Work out the finished part from the listing and answer in its coordinate system (mm). Face numbers are marked on the shaded views. Coordinates: 2 decimals unless noted, no trailing zeros. Order: outer loops, then holes, each group sorted by start corner. A loop starts at its lowest first (then second) coordinate and runs counter-clockwise, first axis right, second up. Notation, with made-up numbers: M 47.5,12 L 59.5,12 A20 ccw 59.5,17 Z; hole C -0.75,86.25 d8. An arc over 180 degrees is marked long. Write item = value, one per line. Start each with the question number.
Q1. Each of these flat-tipped pins is pushed along its axis until it touches: P1, Ø1.5, axis at x = -8, y = 4, coming from the -Z side; P2, Ø3, axis at x = -9.5, y = 2, coming from the -Z side. Where does it stop, or does it pass through?
Q2. Find section A-A on y = 3.5. Give the vertices of the cut face in (x, z) (3 decimals).
Q3. Straight lines are drawn through the part: line 1 along Z through (x, y) = (0, 8.2); line 2 along X through (y, z) = (4, -0.5); line 3 along Z through (x, y) = (0, 0.85). For each, find the intervals that lie inside material, in ascending order.
Q4. Find section D-D on z = 24. Give the vertices of the cut face in (x, y), and give its area (3 significant figures).
Q5. Determine the mould class of the marked faces 1, 2 and 3 for opening direction X: released by +X, released by -X, zero draft, split by the parting line, or undercut.
Q6. Find section B-B on z = 0. Give the vertices of the cut face in (x, y), and give its area (4 significant figures).
Q7. Find section C-C on x = -22.5. Give the vertices of the cut face in (y, z), and give its area (3 significant figures).
Autodesk Inventor part; units mm, degrees
ref_plane "YZ Plane" through (0, 0, 0) normal (1, 0, 0) x (0, 1, 0)
ref_plane "XZ Plane" through (0, 0, 0) normal (0, 1, 0) x (-1, 0, 0)
ref_plane "XY Plane" through (0, 0, 0) normal (0, 0, 1) x (1, 0, 0)
sketch "Náčrt1" plane through (0, 0, 0) normal (0, 1, 0) x (-1, 0, 0)
  line L0 (0, -49) -> (0, 49)
  line L1 (35, -35) -> (-35, -35)
  line L2 (-35, -35) -> (-35, 35)
  line L3 (-35, 35) -> (35, 35)
  line L4 (35, 35) -> (35, -35)
  line L5 (-49, 0) -> (49, 0)
  dimension "d9" = 70
  dimension "d10" = 70
extrude "Vysunutí1" add sketch "Náčrt1" along normal blind 10
fillet "Zaoblení1" radius 6 2 edges at (35, 5, -35) (-35, 5, 35)
fillet "Zaoblení2" radius 34 1 edges at (-35, 5, -35)
sketch "Náčrt2" plane through (0, 10, 0) normal (0, 1, 0) x (1, 0, 0)
  line L0 (0, 49) -> (0, -49)
  line L1 (49, 0) -> (-49, 0)
  point P0 (0, 0)
  point P1 (0, 0)
hole "Díra1" at (0, 10, 0) direction (0, -1, 0) diameter 60.1 depth 7.3 counterbore diameter 62.9 counterbore depth 5.1
sketch "Náčrt3" plane through (0, 2.7, 0) normal (0, 1, 0) x (1, 0, 0)
  line L0 (0, 49) -> (0, -49)
  line L1 (49, 0) -> (-49, 0)
  point P0 (0, 0)
  point P1 (0, 0)
hole "Díra2" at (0, 2.7, 0) direction (0, -1, 0) diameter 58.2 end through all
sketch "Náčrt4" plane through (0, 10, 0) normal (0, 1, 0) x (1, 0, 0)
  arc A0 (-35, -29) -> (-29, -35) centre (-29, -29) ccw
  arc A1 (35, 29) -> (29, 35) centre (29, 29) ccw
  point P0 (0, 0)
hole "Díra3" at (-29, 10, 29) at (29, 10, -29) direction (0, -1, 0) diameter 3.9 end through all
sketch "Náčrt5" plane through (0, 10, 0) normal (0, 1, 0) x (1, 0, 0)
  arc A0 (17.5, -30.3109) -> (30.3109, -17.5) centre (0, 0) ccw
  line L0 (0, 49) -> (0, -49)
  line L1 (49, 0) -> (-49, 0)
  line L2 (0, 0) -> (17.5, -30.3109)
  line L3 (30.3109, -17.5) -> (0, 0)
  dimension "d35" = 35
  dimension "d36" = 30
  dimension "d37" = 30
extrude "Vysunutí2" cut sketch "Náčrt5" against normal up to surface (10 mm away)
fillet "Zaoblení4" radius 20 1 edges at (35, 5, 35)
properties part number "4.L - GM - 01.03" material "LCP plast"
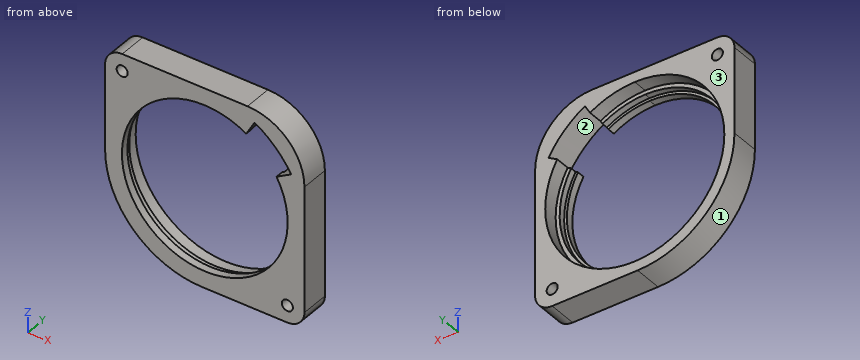
Findings below:
q1.P1 = -34.42
q1.P2 = -34.27
q2.outline = M -35,-1 A34 ccw -1,-35 L 29,-35 A6 ccw 35,-29 L 35,15 A20 ccw 15,35 L -29,35 A6 ccw -35,29 Z; hole C -29,29 d3.9; hole M 15.025,26.024 A30.05 ccw long 26.024,15.025 L 30.311,17.5 A35 ccw 17.5,30.311 Z; hole C 29,-29 d3.9
q3.line_1 = -35 to -31.45, 31.45 to 35
q3.line_2 = -35 to -30.05, 30.05 to 35
q3.line_3 = -35 to -29.1, 29.1 to 35
q4.outline = M -35,0 L -16.46,0 L -16.46,2.7 L -18.08,2.7 L -18.08,4.9 L -20.32,4.9 L -20.32,10 L -35,10 Z; M 25.48,0 L 32.86,0 L 32.86,10 L 25.48,10 Z
q4.area = 236 mm^2
q5.face_1 = released by -X
q5.face_2 = undercut
q5.face_3 = zero draft
q6.outline = M -35,0 L -29.1,0 L -29.1,2.7 L -30.05,2.7 L -30.05,4.9 L -31.45,4.9 L -31.45,10 L -35,10 Z; M 29.1,0 L 35,0 L 35,10 L 31.45,10 L 31.45,4.9 L 30.05,4.9 L 30.05,2.7 L 29.1,2.7 Z
q6.area = 89.85 mm^2
q7.outline = M 0,-27.34 L 10,-27.34 L 10,-21.97 L 4.9,-21.97 L 4.9,-19.92 L 2.7,-19.92 L 2.7,-18.45 L 0,-18.45 Z; M 0,18.45 L 2.7,18.45 L 2.7,19.92 L 4.9,19.92 L 4.9,21.97 L 10,21.97 L 10,35 L 0,35 Z
q7.area = 212 mm^2
